Autodesk Inventor part; units mm, degrees
ref_plane "YZ Plane" through (0, 0, 0) normal (1, 0, 0) x (0, 1, 0)
ref_plane "XZ Plane" through (0, 0, 0) normal (0, 1, 0) x (-1, 0, 0)
ref_plane "XY Plane" through (0, 0, 0) normal (0, 0, 1) x (1, 0, 0)
sketch "Sketch1" plane through (0, 0, 0) normal (0, 0, 1) x (1, 0, 0)
  line L0 (-15, 10) -> (15, 10)
  line L1 (15, 10) -> (15, -10)
  line L2 (15, -10) -> (-15, -10)
  line L3 (-15, -10) -> (-15, 10)
  line L4 (-18.1, 13.1) -> (18.1, 13.1)
  line L5 (18.1, 13.1) -> (18.1, -13.1)
  line L6 (18.1, -13.1) -> (-18.1, -13.1)
  line L7 (-18.1, -13.1) -> (-18.1, 13.1)
  line L8 (16.6, 11.6) -> (-16.6, 11.6)
  line L9 (-16.6, 11.6) -> (-16.6, -11.6)
  line L10 (-16.6, -11.6) -> (16.6, -11.6)
  line L11 (16.6, -11.6) -> (16.6, 11.6)
  line L12 (13.5, 8.5) -> (-13.5, 8.5)
  line L13 (-13.5, 8.5) -> (-13.5, -8.5)
  line L14 (-13.5, -8.5) -> (13.5, -8.5)
  line L15 (13.5, -8.5) -> (13.5, 8.5)
  point P0 (0, 0)
  dimension "d0" = 20
  dimension "d1" = 30
  dimension "d2" = 3.1
  dimension "d3" = 1.6
  dimension "d4" = 1.5
  dimension "d17" = 15
  dimension "d18" = 10
extrude "Extrusion1" add sketch "Sketch1" along normal blind 1 contours L4 L5 L6 L7 | L11 L10 L9 L8
extrude "Extrusion3" add sketch "Sketch1" along normal blind 14 contours L0 L1 L2 L3
sketch "Sketch2" plane through (0, 0, 14) normal (0, 0, 1) x (1, 0, 0)
  line L0 (13.5, 8.5) -> (13.5, -8.5)
  line L1 (13.5, -8.5) -> (-13.5, -8.5)
  line L2 (-13.5, -8.5) -> (-13.5, 8.5)
  line L3 (-13.5, 8.5) -> (13.5, 8.5)
  line L4 (15, 10) -> (-15, 10)
  line L5 (-15, 10) -> (-15, -10)
  line L6 (-15, -10) -> (15, -10)
  line L7 (15, -10) -> (15, 10)
  point P0 (0, 0)
extrude "Extrusion4" add sketch "Sketch2" along normal blind 1.5 contours L0 L1 L2 L3 | L7 L6 L5 L4
fillet "Fillet1" radius 2 8 edges at (-15, 10, 8.25) (-15, -10, 8.25) (15, 10, 8.25) (15, -10, 8.25) (13.5, -8.5, 7) (-13.5, -8.5, 7) (13.5, 8.5, 7) (-13.5, 8.5, 7)
fillet "Fillet1" radius 3 4 edges at (-18.1, -13.1, 0.5) (18.1, -13.1, 0.5) (18.1, 13.1, 0.5) (-18.1, 13.1, 0.5)
fillet "Fillet2" radius 1.5 8 edges at (-14.4142, 9.4142, 15.5) (-15, 0, 15.5) (-14.4142, -9.4142, 15.5) (0, -10, 15.5) (14.4142, -9.4142, 15.5) (15, 0, 15.5) (14.4142, 9.4142, 15.5) (0, 10, 15.5)
sketch "Sketch3" plane through (0, 0, 1) normal (0, 0, 1) x (1, 0, 0)
  arc A0 (-15.1, 13.1) -> (-18.1, 10.1) centre (-15.1, 10.1) ccw
  line L0 (-18.1, 10.1) -> (-18.1, -10.1)
  arc A1 (-18.1, -10.1) -> (-15.1, -13.1) centre (-15.1, -10.1) ccw
  line L1 (-15.1, -13.1) -> (15.1, -13.1)
  arc A2 (15.1, -13.1) -> (18.1, -10.1) centre (15.1, -10.1) ccw
  line L2 (18.1, -10.1) -> (18.1, 10.1)
  arc A3 (18.1, 10.1) -> (15.1, 13.1) centre (15.1, 10.1) ccw
  line L3 (15.1, 13.1) -> (-15.1, 13.1)
  line L4 (15, 8) -> (15, -8)
  arc A4 (13, -10) -> (15, -8) centre (13, -8) ccw
  line L5 (13, -10) -> (-13, -10)
  arc A5 (-15, -8) -> (-13, -10) centre (-13, -8) ccw
  line L6 (-15, -8) -> (-15, 8)
  arc A6 (-13, 10) -> (-15, 8) centre (-13, 8) ccw
  line L7 (-13, 10) -> (13, 10)
  arc A7 (15, 8) -> (13, 10) centre (13, 8) ccw
  line L8 (16.6, -8) -> (16.6, 8)
  arc A8 (16.6, 8) -> (13, 11.6) centre (13, 8) ccw
  line L9 (13, 11.6) -> (-13, 11.6)
  arc A9 (-13, 11.6) -> (-16.6, 8) centre (-13, 8) ccw
  line L10 (-16.6, 8) -> (-16.6, -8)
  arc A10 (-16.6, -8) -> (-13, -11.6) centre (-13, -8) ccw
  line L11 (-13, -11.6) -> (13, -11.6)
  arc A11 (13, -11.6) -> (16.6, -8) centre (13, -8) ccw
  point P0 (0, 0)
  point P1 (15.5456, -10.5456)
  point P2 (0, -11.6)
  point P3 (-15.5456, -10.5456)
  point P4 (-16.6, 0)
  point P5 (16.6, 0)
  point P6 (15.5456, 10.5456)
  point P7 (0, 11.6)
  point P8 (-15.5456, 10.5456)
  dimension "d16" = 1.6
hole "Hole1" at (15.5456, -10.5456, 1) at (0, -11.6, 1) at (-15.5456, -10.5456, 1) at (-16.6, 0, 1) at (16.6, 0, 1) at (15.5456, 10.5456, 1) at (0, 11.6, 1) at (-15.5456, 10.5456, 1) direction (0, 0, -1) diameter 1.6 end through all both
sketch "Sketch4" plane through (-13, 10, 1) normal (0, 1, 0) x (1, 0, 0)
  line L0 (26, -13) -> (0, -13)
  line L1 (26, 0) -> (26, -13)
  line L2 (0, 0) -> (26, 0)
  line L3 (0, -13) -> (0, 0)
  line L4 (24.5, -3.75) -> (24.5, -2.25) construction
  line L5 (25.25, -3.75) -> (25.25, -2.25)
  line L6 (23.75, -2.25) -> (23.75, -3.75)
  arc A0 (23.75, -3.75) -> (25.25, -3.75) centre (24.5, -3.75) ccw
  arc A1 (25.25, -2.25) -> (23.75, -2.25) centre (24.5, -2.25) ccw
  line L7 (25.75, -3.75) -> (25.75, -2.25)
  arc A2 (25.75, -2.25) -> (23.25, -2.25) centre (24.5, -2.25) ccw
  line L8 (23.25, -2.25) -> (23.25, -3.75)
  arc A3 (23.25, -3.75) -> (25.75, -3.75) centre (24.5, -3.75) ccw
  circle A4 centre (24.5, -3.75) radius 0.75
  circle A5 centre (24.5, -2.25) radius 0.75
  point P0 (13, 1)
  point P1 (24.5, -3)
  dimension "d26" = 1.5
  dimension "d27" = 1.5
  dimension "d28" = 1.5
  dimension "d29" = 10
  dimension "d30" = 13
  dimension "d31" = 0.5
extrude "Extrusion5" add sketch "Sketch4" along normal blind 1 contours A3 L8 A2 L7
extrude "Extrusion6" add sketch "Sketch4" along normal blind 10 contours A0 A4 | A5 A1
properties part number "CNCM_ALU_Vibration_module_cover" material "Aluminum 6061"
Geometry: final body of the model. Coordinates: model frame, mm. A direction names the side the tool comes from. Round coordinates to 2 decimals unless told otherwise and drop trailing zeros. Loops run counter-clockwise (first coordinate to the right, second up) from the corner with the lowest first, then second, coordinate; pieces in that order, holes last. Notation, with made-up numbers: (30, -28) -> (36, -28) arc R33 ccw to (36, 6) -> close; hole circle Ø6 at (-24, 4.5). An arc over 180 degrees is marked (long way). Use one line per item in the form item = value.
Item 1: Cut plane D-D on x = -5.5. Output: boundary loops of the cut face in (y, z), then the cut area to 3 significant figures.
Evaluation:
outline = (-13.1, 0) -> (-8.5, 0) -> (-8.5, 14) -> (8.5, 14) -> (8.5, 0) -> (13.1, 0) -> (13.1, 1) -> (10, 1) -> (10, 14) arc R1.5 ccw to (8.5, 15.5) -> (-8.5, 15.5) arc R1.5 ccw to (-10, 14) -> (-10, 1) -> (-13.1, 1) -> close
area = 77.2 mm2
Item 2: Material intervals for probe 1 along X at (y, z) = (0, 0.55); probe 2 along Y at (x, z) = (-8, 10.5); probe 3 along X at (y, z) = (4, 5), sorted ascending.
Evaluation:
probe_1 = -18.1 to -17.4, -15.8 to -13.5, 13.5 to 15.8, 17.4 to 18.1
probe_2 = -10 to -8.5, 8.5 to 10
probe_3 = -15 to -13.5, 13.5 to 15
Item 3: Contact query for flat-ended pins moving along their axis: pin 1 Ø2 at (x, z) = (0.5, 5.5) entering from +Y; pin 2 Ø1.1 at (x, z) = (-5.5, 0.5) entering from +Y; pin 3 Ø1.4 at (x, y) = (-16.6, 0) entering from +Z; pin 4 Ø1.5 at (x, z) = (-1, 4) entering from -Y. Output: stop coordinate, or through.
Evaluation:
pin_1 = 10
pin_2 = 13.1
pin_3 = through
pin_4 = -10
Item 4: Cut plane C-C on x = 0. Output: boundary loops of the cut face in (y, z), then the cut area to 3 significant figures.
Evaluation:
outline = (-13.1, 0) -> (-12.4, 0) -> (-12.4, 1) -> (-13.1, 1) -> close; (-10.8, 0) -> (-8.5, 0) -> (-8.5, 14) -> (8.5, 14) -> (8.5, 0) -> (10.8, 0) -> (10.8, 1) -> (10, 1) -> (10, 14) arc R1.5 ccw to (8.5, 15.5) -> (-8.5, 15.5) arc R1.5 ccw to (-10, 14) -> (-10, 1) -> (-10.8, 1) -> close; (12.4, 0) -> (13.1, 0) -> (13.1, 1) -> (12.4, 1) -> close
area = 74.0 mm2
Item 5: Access query for faces 1 (the flat face through (0, -8.5, 7)), 2 (the flat face through (10.6, 11, 4)), 3 (the cylindrical face through (14.4, 9.43, 7.41)), 4 (the cylindrical face through (-0.18, 9.55, 15.07)), 5 (the cylindrical face through (17.2, -12.24, 0.51)). Directions: +Z, -Z, +X, -X, +Y, -Y. A direction counts if a zero-diameter tool reaches every point of the face in a straight line with its end or side. Return the directions, or none.
Evaluation:
face_1 = -Z
face_2 = +Y
face_3 = +Z, +X, +Y
face_4 = +Z, +X, -X, +Y
face_5 = +Z, -Z, +X, -Y
Item 6: Draft query along X for faces 6 (the flat face through (15, 0, 7)), 7 (the cylindrical face through (-14.43, -9.4, 7.59)), 8 (the cylindrical face through (-15.82, 0.17, 0.49)). Return one class per face: released by +X, released by -X, zero draft, split by the parting line, or undercut.
Evaluation:
face_6 = released by +X
face_7 = released by -X
face_8 = undercut
Item 7: Cut plane A-A on y = 0. Output: boundary loops of the cut face in (x, z), then the cut area to 3 significant figures.
Evaluation:
outline = (-18.1, 0) -> (-17.4, 0) -> (-17.4, 1) -> (-18.1, 1) -> close; (-15.8, 0) -> (-13.5, 0) -> (-13.5, 14) -> (13.5, 14) -> (13.5, 0) -> (15.8, 0) -> (15.8, 1) -> (15, 1) -> (15, 14) arc R1.5 ccw to (13.5, 15.5) -> (-13.5, 15.5) arc R1.5 ccw to (-15, 14) -> (-15, 1) -> (-15.8, 1) -> close; (17.4, 0) -> (18.1, 0) -> (18.1, 1) -> (17.4, 1) -> close
area = 89.0 mm2
Item 8: Cut plane B-B on z = 8.5. Output: boundary loops of the cut face in (x, y), then the cut area to 3 significant figures.
Evaluation:
outline = (-15, -8) arc R2 ccw to (-13, -10) -> (13, -10) arc R2 ccw to (15, -8) -> (15, 8) arc R2 ccw to (13, 10) -> (-13, 10) arc R2 ccw to (-15, 8) -> close; hole (-13.5, -6.5) arc R2 ccw to (-11.5, -8.5) -> (11.5, -8.5) arc R2 ccw to (13.5, -6.5) -> (13.5, 6.5) arc R2 ccw to (11.5, 8.5) -> (-11.5, 8.5) arc R2 ccw to (-13.5, 6.5) -> close
area = 141 mm2
